Geometry check sheet. Reference: the model listing, model coordinates, mm. Face numbers are marked on the shaded views. A direction names the side the tool comes from. Give positions to 0.01 mm unless a question says otherwise; leave off trailing zeros. Write each loop counter-clockwise with the first axis right and the second up, starting at its lowest first coordinate (ties: lowest second). Pieces come first, ordered by that corner, then holes. Notation, with made-up numbers: (-31, 35) - (11, 35) arc R12 cw to (11, 48) - close; hole circle Ø1 at (21.5, 44.25). An arc over 180 degrees is marked (long way). Use a Markdown table: item, result.
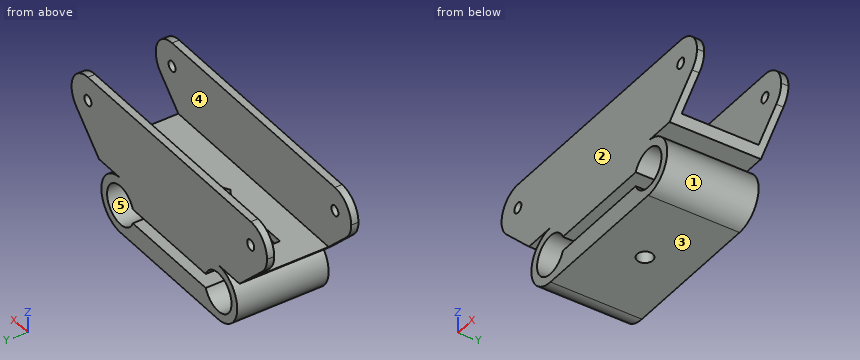
```python
from build123d import *

# Parameters (mm, degrees)
F2_DEPTH  = 60
F4_DEPTH  = 19
F0_R      = 2.15
F5_DEPTH  = 30.3
F6_R      = 10
F7_R      = 3.3
F8_DEPTH  = 29.5
F10_DEPTH = 6
F9_W      = 12
F9_H      = 8
F11_DEPTH = 3
F13_DEPTH = 25


with BuildPart() as f2:
    # F1 (on Right) → F2 (new body, symmetric)
    with BuildSketch(Plane.YZ):
        Polygon((16, 0), (-16, 0), (-16, 28), (-19, 28), (-19, -3), (19, -3), (19, 28), (16, 28), align=None)
    extrude(amount=F2_DEPTH, both=True)

    # F3 (on Front) → F4 (join, symmetric)
    with BuildSketch(Plane.XZ):
        with BuildLine():
            Line((0, -3), (-30, -3))
            ThreePointArc((-30, -3), (-41.7, -14.7), (-30, -26.4))
            Line((-30, -26.4), (0, -26.4))
            Line((0, -26.4), (30, -26.4))
            ThreePointArc((30, -26.4), (41.7, -14.7), (30, -3))
            Line((30, -3), (0, -3))
        make_face()
        with BuildLine():
            ThreePointArc((-22.368486, -17.7), (-38.2, -14.7), (-22.368486, -11.7))
            Line((-22.368486, -11.7), (0, -11.7))
            Line((0, -11.7), (22.368486, -11.7))
            ThreePointArc((22.368486, -11.7), (38.2, -14.7), (22.368486, -17.7))
            Line((22.368486, -17.7), (0, -17.7))
            Line((0, -17.7), (-22.368486, -17.7))
        make_face(mode=Mode.SUBTRACT)
    extrude(amount=F4_DEPTH, both=True)

    # F0 (on Front) → F5 (cut, symmetric)
    with BuildSketch(Plane.XZ):
        with Locations((-50, 18)):
            Circle(F0_R)
        with Locations((50, 18)):
            Circle(F0_R)
    extrude(amount=F5_DEPTH, both=True, mode=Mode.SUBTRACT)

    # F6
    f6_edges = [f2.edges().sort_by_distance(p)[0] for p in [
        (-60, -17.5, 28),
        (-60, 17.5, 28),
        (60, 17.5, 28),
        (60, -17.5, 28),
    ]]
    fillet(f6_edges, radius=F6_R)

    # F7 (on Top) → F8 (cut, symmetric)
    with BuildSketch(Plane.XY):
        Circle(F7_R)
    extrude(amount=F8_DEPTH, both=True, mode=Mode.SUBTRACT)

    # F9 (on Top) → F10 (cut)
    with BuildSketch(Plane.XY):
        Polygon((5.5, -3.175426), (5.5, 3.175426), (0, 6.350853), (-5.5, 3.175426), (-5.5, -3.175426), (0, -6.350853), align=None)
    extrude(amount=-F10_DEPTH, mode=Mode.SUBTRACT)

    # F9 (on Top) → F11 (cut)
    with BuildSketch(Plane.XY):
        with Locations((-28, 0)):
            Rectangle(F9_W, F9_H)
        with Locations((28, 0)):
            Rectangle(F9_W, F9_H)
    extrude(amount=-F11_DEPTH, mode=Mode.SUBTRACT)

    # F12 (on Front) → F13 (cut, symmetric)
    with BuildSketch(Plane.XZ):
        with BuildLine():
            Line((56.966549, 10.825936), (43.140613, -3))
            Line((43.140613, -3), (66.425517, -3))
            Line((66.425517, -3), (66.425517, 22.940923))
            Line((66.425517, 22.940923), (58.694095, 22.940923))
            ThreePointArc((58.694095, 22.940923), (59.899857, 16.588322), (56.966549, 10.825936))
        make_face()
        with BuildLine():
            ThreePointArc((-56.966549, 10.825936), (-59.899857, 16.588322), (-58.694095, 22.940923))
            Line((-58.694095, 22.940923), (-66.425517, 22.940923))
            Line((-66.425517, 22.940923), (-66.425517, -3))
            Line((-66.425517, -3), (-43.140613, -3))
            Line((-43.140613, -3), (-56.966549, 10.825936))
        make_face()
    extrude(amount=F13_DEPTH, both=True, mode=Mode.SUBTRACT)


solid = f2.part
```
1) Material ranges on L1, parallel to Y at x = 39.5, z = 11.5; L2, parallel to X at y = -15.5, z = -11.5; L3, parallel to X at y = 5.5, z = -14.7, recorded low to high. Write a range as from..to.
Working result:
| item | result |
|---|---|
| L1 | y = -19..-16, 16..19 |
| L2 | x = -41.25..-37.55, -22.45..22.45, 37.55..41.25 |
| L3 | x = -41.7..-38.2, 38.2..41.7 |
2) Section check A-A on z = -14.7. Record the boundary of the cut face in (x, y).
Working result:
| item | result |
|---|---|
| outline | (-41.7, -19) - (-38.2, -19) - (-38.2, 19) - (-41.7, 19) - close; (38.2, -19) - (41.7, -19) - (41.7, 19) - (38.2, 19) - close |
3) Mould release check, pull along Z, two halves, no side actions. Record for the marked faces 1, 2 and 3: pulls with the +Z half, pulls with the -Z half, needs draft (parallel to the pull), parting line crosses it, or undercut.
Working result:
| item | result |
|---|---|
| face 1 | undercut |
| face 2 | needs draft |
| face 3 | pulls with the -Z half |
4) Section check B-B on x = 18.5. Record the boundary of the cut face in (y, z).
Working result:
| item | result |
|---|---|
| outline | (-19, -26.4) - (19, -26.4) - (19, -17.7) - (-19, -17.7) - close; (-19, -11.7) - (19, -11.7) - (19, 28) - (16, 28) - (16, 0) - (-16, 0) - (-16, 28) - (-19, 28) - close |
5) Set-up check for the marked faces 4 and 5: record each of +Z, -Z, +X, -X, +Y, -Y from which the full face is reachable in a straight line by a thin tool's end or side.
Working result:
| item | result |
|---|---|
| face 4 | +Z, +X, -X |
| face 5 | +Y, -Y |
6) Section check C-C on x = 32. Record the boundary of the cut face in (y, z).
Working result:
| item | result |
|---|---|
| outline | (-19, -26.23) - (19, -26.23) - (19, -22.65) - (-19, -22.65) - close; (-19, -6.75) - (19, -6.75) - (19, -3.17) - (-19, -3.17) - close; (-19, -3) - (-4, -3) - (-4, 0) - (-16, 0) - (-16, 28) - (-19, 28) - close; (4, -3) - (19, -3) - (19, 28) - (16, 28) - (16, 0) - (4, 0) - close |
7) Section check D-D on z = 4. Record the boundary of the cut face in (x, y), then the cut area to 3 significant figures.
Working result:
| item | result |
|---|---|
| outline | (-50.14, -19) - (50.14, -19) - (50.14, -16) - (-50.14, -16) - close; (-50.14, 16) - (50.14, 16) - (50.14, 19) - (-50.14, 19) - close |
| area | 602 mm² |
8) Depth check by flat-ended pin: P1, Ø9.5, axis at x = 0, y = 4, coming from the +Z side; P2, Ø10.5, axis at x = -36.5, y = 0, coming from the -Z side; P3, Ø3.5, axis at y = 2, z = -1.5, coming from the -X side. Enter the tip coordinate at first touch or a pass-through.
Working result:
| item | result |
|---|---|
| P1 | stops at z = 0 |
| P2 | stops at z = -26.33 |
| P3 | stops at x = -46.14 |
